Build history of the part. All positions in model axes, mm. Face numbers are marked on the shaded views. Round coordinates to 2 decimals unless told otherwise and drop trailing zeros. Put each result on its own line as item: value. Start each with the question number.
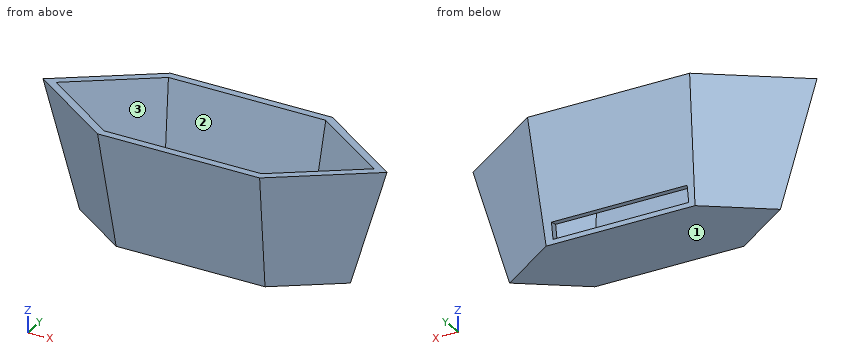
from build123d import *

# Parameters (mm, degrees)
F1_DEPTH = 40
F1_TAPER = -10
F2_T     = -2.5
F3_W     = 45.5802325159
F3_H     = 5.3462651558
F4_DEPTH = 5


with BuildPart() as f1:
    # F0 (on Top) → F1 (new body)
    with BuildSketch(Plane.XY):
        Polygon((24.8156337307, 0), (0, 0), (-25.1843662693, 0), (-45.6631673765, -14.3394109088), (-25.1843662693, -28.6788218176), (24.8156337307, -28.6788218176), (45.294434838, -14.3394109088), align=None)
    extrude(amount=F1_DEPTH, taper=F1_TAPER)

    # F2
    f2_openings = [f1.faces().sort_by_distance(p)[0] for p in [
        (-0.184366, -14.339411, 40),
    ]]
    offset(amount=F2_T, openings=f2_openings)

    # F3 (on face) → F4 (cut)
    with BuildSketch(Plane(origin=(0, 0, 0), x_dir=(-1, 0, 0), z_dir=(0, 0.984807753, -0.1736481777))):
        with Locations((0.4246877506, 4.1624491569)):
            Rectangle(F3_W, F3_H)
    extrude(amount=-F4_DEPTH, mode=Mode.SUBTRACT)


solid = f1.part
Item 1: Drop flat-ended pins along their axis: pin 1 Ø12 at (x, y) = (1.5, -19) entering from +Z; pin 2 Ø5 at (y, z) = (-4, 8) entering from -X; pin 3 Ø2 at (y, z) = (-28.5, 14.5) entering from -X. Give the stop position or say it passes through.
Item 2: Drill centre lines: probe 1 along Y at (x, z) = (28, 7.5); probe 2 along Y at (x, z) = (11, 15); probe 3 along Z at (x, y) = (-19.5, -20.5). Where is each one in solid material? Low to high. Write a range as [from, to].
Item 3: Two-plate mould, pull along X, no slides. Class the marked faces 1, 2 and 3: pulls with the +X half, pulls with the -X half, needs draft (parallel to the pull), parting line crosses it, or undercut.
Computed values:
1. pin 1: stops at z = 2.5
1. pin 2: stops at x = -37.01
1. pin 3: stops at x = -31.36
2. probe 1: y = [-28.06, -24.96], [-3.71, -0.62]
2. probe 2: y = [-31.32, -28.79], [0.11, 2.64]
2. probe 3: z = [0, 2.5]
3. face 1: needs draft
3. face 2: undercut
3. face 3: undercut
